CAD build for the part. Positions are in the model's coordinates, mm. A direction names the side the tool comes from. Coordinates: 2 decimals unless noted, no trailing zeros. Loops run counter-clockwise (first coordinate to the right, second up) from the corner with the lowest first, then second, coordinate; pieces in that order, holes last. Notation, with made-up numbers: M 38,73 L 50,73 A18 ccw 50,96 Z; hole C -32.75,-12 d11. An arc over 180 degrees is marked long. Answer as a JSON object with one key per item and string values. Group by question number.
Autodesk Inventor part; units mm, degrees
ref_plane "YZ Plane" through (0, 0, 0) normal (1, 0, 0) x (0, 1, 0)
ref_plane "XZ Plane" through (0, 0, 0) normal (0, 1, 0) x (-1, 0, 0)
ref_plane "XY Plane" through (0, 0, 0) normal (0, 0, 1) x (1, 0, 0)
sketch "Sketch1" plane through (0, 0, 0) normal (0, 0, 1) x (1, 0, 0)
  line L0 (0, 0) -> (0, 38.1)
  line L1 (0, 38.1) -> (12.7, 38.1)
  line L2 (12.7, 38.1) -> (12.7, 12.7)
  line L3 (12.7, 12.7) -> (38.1, 12.7)
  line L4 (38.1, 12.7) -> (38.1, 0)
  line L5 (38.1, 0) -> (0, 0)
  dimension "d0" = 38.1
  dimension "d1" = 12.7
  dimension "d2" = 25.4
  dimension "d3" = 25.4
extrude "Extrusion1" add sketch "Sketch1" along normal blind 38.1
chamfer "Chamfer1" distance 3.175 angle 45 1 edges at (12.7, 38.1, 19.05)
chamfer "Chamfer2" distance 3.175 angle 45 2 edges at (12.7, 12.7, 19.05) (38.1, 12.7, 19.05)
properties part number "ChamferPart"
Item 1: Tool access for faces 1 (the flat face through (38.1, 5, 19)), 2 (the flat face through (12.7, 26, 19)): list every direction of +Z, -Z, +X, -X, +Y, -Y with a clear straight run to the whole face (end or side of a thin tool).
Item 2: Slice it at B-B, the plane y = 25. Write the cut outline in (x, z), then the cut area to 3 significant figures.
Item 3: Drill centre lines: L1, parallel to X at y = 32, z = 22.5; L2, parallel to X at y = 12, z = 9 (3 decimals). Where is each one in solid material? Low to high. Write a range as from..to.
Item 4: Pin check, flat tips, straight feed: pin 1 (8 mm diameter, centred on y = 18.5, z = 33.5, fed in from +X) (3 decimals); pin 2 (6 mm diameter, centred on x = 29.5, z = 12.5, fed in from +Y); pin 3 (15 mm diameter, centred on y = 29, z = 13, fed in from +X). Stop position of each tip, or through.
Item 5: Slice it at A-A, the plane z = 24. Write the cut outline in (x, y) (3 decimals), then the cut area to 3 significant figures.
Computed:
{
 "1": {"face 1": "+Z, -Z, +X, +Y, -Y", "face 2": "+Z, -Z, +X, +Y"},
 "2": {"outline": "M 0,0 L 12.7,0 L 12.7,38.1 L 0,38.1 Z", "area": "484 mm2"},
 "3": {"L1": "0..12.7", "L2": "0..35.625"},
 "4": {"pin 1": "x = 14.075", "pin 2": "y = 12.7", "pin 3": "x = 12.7"},
 "5": {"outline": "M 0,0 L 38.1,0 L 38.1,9.525 L 34.925,12.7 L 15.875,12.7 L 12.7,15.875 L 12.7,34.925 L 9.525,38.1 L 0,38.1 Z", "area": "801 mm2"}
}
